Verification items for the finished model (mm, model axes). Face numbers are marked on the shaded views. A direction names the side the tool comes from. Coordinates: 2 decimals unless noted, no trailing zeros. Write each loop counter-clockwise with the first axis right and the second up, starting at its lowest first coordinate (ties: lowest second). Pieces come first, ordered by that corner, then holes. Notation, with made-up numbers: (10.25, 71.25) - (14.25, 71.25) arc R32 ccw to (14.25, 99.25) - close; hole circle Ø7 at (37.5, 68.5). An arc over 180 degrees is marked (long way). Use one line per item in the form item = value. Start each with the question number.
(1) Sectioned sample at A-A (x = 12.5). Record the cut outline in (y, z), and give its area (3 significant figures).
(2) Sectioned sample at C-C (y = 36.25). Record the cut outline in (x, z).
(3) Material ranges on line 1 (X direction, y = 36.25, z = -3.5); line 2 (Y direction, x = 0, z = 1.2); line 3 (Y direction, x = -13, z = -1.75), recorded low to high. Write a range as [from, to].
(4) Sectioned sample at D-D (y = -1.5). Record the cut outline in (x, z).
(5) Sectioned sample at B-B (z = -2). Record the cut outline in (x, y).
(6) Tool access check on the marked faces 1 and 2. Record the directions out of +Z, -Z, +X, -X, +Y, -Y that give a thin tool (end or side, any length) a straight path to the whole face; none if there is none.
(7) Gauge pin test, flat ends, axial feed: pin 1 Ø3 at (x, z) = (-23.5, -11.5) entering from +Y; pin 2 Ø5 at (x, y) = (23.5, -15.5) entering from -Z; pin 3 Ø5 at (x, y) = (12.5, 36.25) entering from -Z. Record the tip position at first contact, or that the pin passes through.
from build123d import *

# Parameters (mm, degrees)
CROQUIS1_W              = 64.5
CROQUIS1_H              = 53.5
SALIENTE_EXTRUIR1_DEPTH = 2
CROQUIS2_W              = 64.5
CROQUIS2_H              = 5
SALIENTE_EXTRUIR2_DEPTH = 5
CROQUIS3_W              = 64.5
CROQUIS3_H              = 2
SALIENTE_EXTRUIR3_DEPTH = 20
CROQUIS5_R              = 3
CORTAR_EXTRUIR1_DEPTH   = 20
CROQUIS7_W              = 5
CROQUIS7_H              = 5.397784026
CORTAR_EXTRUIR3_DEPTH   = 73.634788497
CROQUIS8_W              = 2
CROQUIS8_H              = 10
CROQUIS8_H_2            = 5
CROQUIS8_W_2            = 5
SALIENTE_EXTRUIR4_DEPTH = 64.5
CROQUIS9_R              = 1.95
CORTAR_EXTRUIR4_DEPTH   = 53.598716714


with BuildPart() as part:
    # Croquis1 → Saliente-Extruir1 (new body)
    with BuildSketch(Plane.XY):
        Rectangle(CROQUIS1_W, CROQUIS1_H)
    extrude(amount=SALIENTE_EXTRUIR1_DEPTH)

    # Croquis2 → Saliente-Extruir2 (add)
    with BuildSketch(Plane(origin=(0, 0, 0), x_dir=(-1, 0, 0), z_dir=(0, 0, -1))):
        with Locations((0, 24.25)):
            Rectangle(CROQUIS2_W, CROQUIS2_H)
    extrude(amount=SALIENTE_EXTRUIR2_DEPTH)

    # Croquis3 → Saliente-Extruir3 (add)
    with BuildSketch(Plane(origin=(0, 0, 0), x_dir=(-1, 0, 0), z_dir=(0, 0, -1))):
        with Locations((0, -25.75)):
            Rectangle(CROQUIS3_W, CROQUIS3_H)
    extrude(amount=SALIENTE_EXTRUIR3_DEPTH)

    # Croquis5 → Cortar-Extruir1 (cut)
    with BuildSketch(Plane(origin=(0, 0, 0), x_dir=(-1, 0, 0), z_dir=(0, 0, -1))):
        with Locations((0, -1.5)):
            Circle(CROQUIS5_R)
    extrude(amount=-CORTAR_EXTRUIR1_DEPTH, mode=Mode.SUBTRACT)

    # Croquis7 → Cortar-Extruir3 (cut, through all)
    with BuildSketch(Plane(origin=(32.25, 0, 0), x_dir=(0, 0, -1), z_dir=(1, 0, 0))):
        with Locations((2.5, 24.051107987)):
            Rectangle(CROQUIS7_W, CROQUIS7_H)
    extrude(amount=-CORTAR_EXTRUIR3_DEPTH, mode=Mode.SUBTRACT)

    # Croquis8 → Saliente-Extruir4 (add, through all)
    with BuildSketch(Plane(origin=(32.25, 0, 0), x_dir=(0, 0, -1), z_dir=(1, 0, 0))):
        with Locations((-1, 28.75)):
            Rectangle(CROQUIS8_W, CROQUIS8_H)
        with Locations((-1, 36.25)):
            Rectangle(CROQUIS8_W, CROQUIS8_H_2)
        with Locations((2.5, 36.25)):
            Rectangle(CROQUIS8_W_2, CROQUIS8_H_2)
    extrude(amount=-SALIENTE_EXTRUIR4_DEPTH)

    # Croquis9 → Cortar-Extruir4 (cut, through all)
    with BuildSketch(Plane(origin=(0, 0, -5), x_dir=(-1, 0, 0), z_dir=(0, 0, -1))):
        with Locations(Location((-12.5, 36.25, 0), (0, 0, 90))):
            Circle(CROQUIS9_R)
        with Locations(Location((12.5, 36.25, 0), (0, 0, 270))):
            Circle(CROQUIS9_R)
    extrude(amount=-CORTAR_EXTRUIR4_DEPTH, mode=Mode.SUBTRACT)


solid = part.part
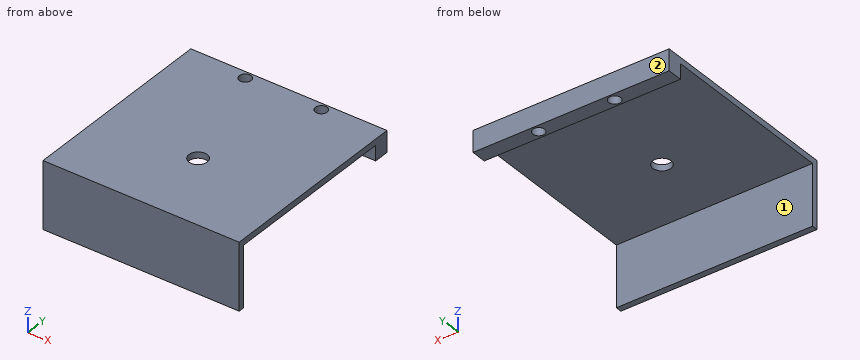
Answers below:
q1.outline = (-26.75, -20) - (-24.75, -20) - (-24.75, 0) - (33.75, 0) - (33.75, -5) - (34.3, -5) - (34.3, 2) - (-26.75, 2) - close; (38.2, -5) - (38.75, -5) - (38.75, 2) - (38.2, 2) - close
q1.area = 169 mm2
q2.outline = (-32.25, -5) - (-14.45, -5) - (-14.45, 2) - (-32.25, 2) - close; (-10.55, -5) - (10.55, -5) - (10.55, 2) - (-10.55, 2) - close; (14.45, -5) - (32.25, -5) - (32.25, 2) - (14.45, 2) - close
q3.line_1 = [-32.25, -14.45], [-10.55, 10.55], [14.45, 32.25]
q3.line_2 = [-26.75, -4.5], [1.5, 38.75]
q3.line_3 = [-26.75, -24.75], [33.75, 34.37], [38.13, 38.75]
q4.outline = (-32.25, 0) - (-3, 0) - (-3, 2) - (-32.25, 2) - close; (3, 0) - (32.25, 0) - (32.25, 2) - (3, 2) - close
q5.outline = (-32.25, -26.75) - (32.25, -26.75) - (32.25, -24.75) - (-32.25, -24.75) - close; (-32.25, 33.75) - (32.25, 33.75) - (32.25, 38.75) - (-32.25, 38.75) - close; hole circle Ø3.9 at (-12.5, 36.25); hole circle Ø3.9 at (12.5, 36.25)
q6.face_1 = -Z, +X, -X
q6.face_2 = +Z, -Z, +X, -X, +Y
q7.pin_1 = -24.75
q7.pin_2 = 0
q7.pin_3 = -5
